```python
from build123d import *

# Parameters (mm, degrees)
SALIENTE_EXTRUIR1_DEPTH = 5
CROQUIS2_R              = 12.7
CORTAR_EXTRUIR1_DEPTH   = 10
CORTAR_EXTRUIR2_DEPTH   = 10


with BuildPart() as part:
    # Croquis1 → Saliente-Extruir1 (new body)
    with BuildSketch(Plane.XY):
        with BuildLine():
            Line((0, 100), (0, 0))
            Line((0, 0), (100, 0))
            ThreePointArc((100, 0), (70.710678119, 70.710678119), (0, 100))
        make_face()
    extrude(amount=SALIENTE_EXTRUIR1_DEPTH)

    # Croquis2 → Cortar-Extruir1 (cut)
    with BuildSketch(Plane.XY.offset(5)):
        with Locations((20, 32.5)):
            Circle(CROQUIS2_R)
    extrude(amount=-CORTAR_EXTRUIR1_DEPTH, mode=Mode.SUBTRACT)

    # Croquis3 → Cortar-Extruir2 (cut)
    with BuildSketch(Plane.XY.offset(5)):
        with BuildLine():
            Line((8.78881249, 48.063247001), (8.78881249, 89.15262579))
            Line((8.78881249, 89.15262579), (13.826190337, 78.875233565))
            ThreePointArc((13.826190337, 78.875233565), (19.806584532, 82.16151857), (24.282169152, 87.312627788))
            ThreePointArc((24.282169152, 87.312627788), (26.07485748, 86.878519508), (27.856038853, 86.399380324))
            Line((27.856038853, 86.399380324), (30.697722068, 76.655190323))
            ThreePointArc((30.697722068, 76.655190323), (36.801955218, 77.531012101), (42.084756772, 80.712322191))
            ThreePointArc((42.084756772, 80.712322191), (65.921457687, 60.654047665), (79.258334665, 32.5))
            Line((79.258334665, 32.5), (39.180859798, 32.5))
            ThreePointArc((39.180859798, 32.5), (28.742573042, 49.572574475), (8.78881249, 48.063247001))
        make_face()
    extrude(amount=-CORTAR_EXTRUIR2_DEPTH, mode=Mode.SUBTRACT)


solid = part.part
```
Check sheet for the modelled part. Datum: model origin and axes. Units: mm. A direction names the side the tool comes from. Coordinates: 2 decimals unless noted, no trailing zeros. Order: outer loops, then holes, each group sorted by start corner. A loop starts at its lowest first (then second) coordinate and runs counter-clockwise, first axis right, second up. Notation, with made-up numbers: (81.5, 48.25) -> (114.5, 48.25) arc R22 cw to (114.5, 69.25) -> close; hole circle Ø5 at (59, 86). An arc over 180 degrees is marked (long way). Write item = value, one per line. Start each with the question number.
1) Cross-section at C-C (x = 10). Enter the section's corners in (y, z), then the cut area to 3 significant figures.
2) Material ranges on L1, parallel to Y at x = 20, z = 1.9; L2, parallel to X at y = 44, z = 4.7; L3, parallel to Y at x = 26, z = 2.7, recorded low to high.
3) Mould release check, pull along Y, two halves, no side actions. Record for faces 3 (the flat face through (49, 0, 2)), 4 (the flat face through (38, 28, 5)), 5 (the flat face through (60, 32.5, 3)): +Y half, -Y half, draft (parallel to the pull), parting line (faces both ways), or undercut.
4) Cross-section at A-A (z = 1.3). Enter the section's corners in (x, y).
5) Access from +Z, -Z, +X, -X, +Y, -Y to the whole of each face (thin tool, end or side, straight path). Record for faces 1 (the cylindrical face through (19.73, 82.1, 2.54)), 2 (the flat face through (38, 28, 0)).
6) Cross-section at B-B (y = 69). Enter the section's corners in (x, z), then the cut area to 3 significant figures.
7) Cross-section at D-D (x = 55). Enter the section's corners in (y, z), then the cut area to 3 significant figures.
8) Go/stop test with flat-tipped pins: P1, Ø3, axis at x = 71, y = 19.5, coming from the -Z side; P2, Ø3, axis at x = 75, z = 1, coming from the +Y side; P3, Ø2.5, axis at y = 61.5, z = 2, coming from the +X side; P4, Ø2, axis at y = 38, z = 4, coming from the +X side. Record where each tip stops, or that it passes through.
Ans:
q1.outline = (0, 0) -> (24.67, 0) -> (24.67, 5) -> (0, 5) -> close; (40.33, 0) -> (48.87, 0) -> (48.87, 5) -> (40.33, 5) -> close; (86.68, 0) -> (99.5, 0) -> (99.5, 5) -> (86.68, 5) -> close
q1.area = 230 mm²
q2.L1 = 0 to 19.8, 45.2 to 51.68, 82.32 to 97.98
q2.L2 = 0 to 14.61, 25.39 to 35.35, 75.57 to 89.8
q2.L3 = 0 to 21.31, 43.69 to 50.72, 86.9 to 96.56
q3.face_3 = -Y half
q3.face_4 = draft
q3.face_5 = undercut
q4.outline = (0, 0) -> (100, 0) arc R100 ccw to (0, 100) -> close; hole circle Ø25.4 at (20, 32.5); hole (8.79, 48.06) arc R19.18 cw to (39.18, 32.5) -> (79.26, 32.5) arc R73.2 ccw to (42.08, 80.71) arc R15.54 cw to (30.7, 76.66) -> (27.86, 86.4) arc R73.2 ccw to (24.28, 87.31) arc R19.43 cw to (13.83, 78.88) -> (8.79, 89.15) -> close
q5.face_1 = +Z, -Z
q5.face_2 = -Z, +X, -X, +Y, -Y
q6.outline = (0, 0) -> (8.79, 0) -> (8.79, 5) -> (0, 5) -> close; (58.4, 0) -> (72.38, 0) -> (72.38, 5) -> (58.4, 5) -> close
q6.area = 114 mm²
q7.outline = (0, 0) -> (32.5, 0) -> (32.5, 5) -> (0, 5) -> close; (72.04, 0) -> (83.52, 0) -> (83.52, 5) -> (72.04, 5) -> close
q7.area = 220 mm²
q8.P1 = 0
q8.P2 = 67.81
q8.P3 = 79.81
q8.P4 = 92.9
